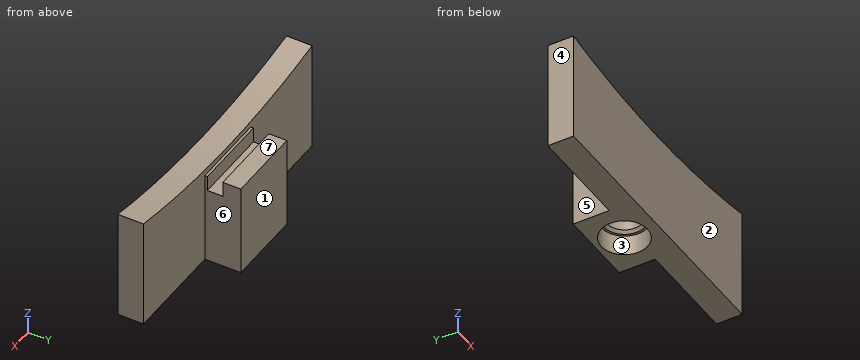
from build123d import *

# Parameters (mm, degrees)
BOSS_EXTRUDE1_DEPTH             = 5
SKETCH4_W                       = 15
SKETCH4_H                       = 18
BOSS_EXTRUDE2_DEPTH             = 0.5
SKETCH5_W                       = 15
SKETCH5_H                       = 15
BOSS_EXTRUDE3_DEPTH             = 3
SKETCH6_W                       = 15
SKETCH6_H                       = 18
BOSS_EXTRUDE4_DEPTH             = 3.5
SKETCH9_R                       = 4.5
CUT_EXTRUDE1_DEPTH              = 4
M8X1_0_TAPPED_HOLE1_D           = 7
M8X1_0_TAPPED_HOLE1_DEPTH       = 8
M8X1_0_TAPPED_HOLE1_CSINK_D     = 8.05
M8X1_0_TAPPED_HOLE1_CSINK_ANGLE = 90
M8X1_0_TAPPED_HOLE1_TIP         = 2.103012167


with BuildPart() as part:
    # Sketch1 → Boss-Extrude1 (new body)
    with BuildSketch(Plane(origin=(0, 0, 0), x_dir=(1, 0, 0), z_dir=(0, 1, 0))):
        with BuildLine():
            Line((0, 9.997621031), (0, 31.54))
            Line((0, 31.54), (55, 31.54))
            Line((55, 31.54), (55, 9.997621031))
            ThreePointArc((55, 9.997621031), (27.5, 12.54), (0, 9.997621031))
        make_face()
    extrude(amount=BOSS_EXTRUDE1_DEPTH)

    # Sketch4 → Boss-Extrude2 (add)
    with BuildSketch(Plane(origin=(0, 5, 0), x_dir=(1, 0, 0), z_dir=(0, 1, 0))):
        with Locations((27.5, 22.54)):
            Rectangle(SKETCH4_W, SKETCH4_H)
    extrude(amount=BOSS_EXTRUDE2_DEPTH)

    # Sketch5 → Boss-Extrude3 (add)
    with BuildSketch(Plane(origin=(0, 5.5, 0), x_dir=(1, 0, 0), z_dir=(0, 1, 0))):
        with Locations((27.5, 24.04)):
            Rectangle(SKETCH5_W, SKETCH5_H)
    extrude(amount=BOSS_EXTRUDE3_DEPTH)

    # Sketch6 → Boss-Extrude4 (add)
    with BuildSketch(Plane(origin=(0, 8.5, 0), x_dir=(1, 0, 0), z_dir=(0, 1, 0))):
        with Locations((27.5, 22.54)):
            Rectangle(SKETCH6_W, SKETCH6_H)
    extrude(amount=BOSS_EXTRUDE4_DEPTH)

    # Sketch9 → Cut-Extrude1 (cut)
    with BuildSketch(Plane(origin=(0, 0, -31.54), x_dir=(-1, 0, 0), z_dir=(0, 0, -1))):
        with Locations((-27.5, 6.5)):
            Circle(SKETCH9_R)
    extrude(amount=-CUT_EXTRUDE1_DEPTH, mode=Mode.SUBTRACT)

    # M8x1.0 Tapped Hole1
    with Locations(Plane(origin=(0, 0, -27.54), x_dir=(-1, 0, 0), z_dir=(0, 0, -1))):
        with Locations((-27.5, 6.5)):
            CounterSinkHole(M8X1_0_TAPPED_HOLE1_D / 2, M8X1_0_TAPPED_HOLE1_CSINK_D / 2, depth=M8X1_0_TAPPED_HOLE1_DEPTH, counter_sink_angle=M8X1_0_TAPPED_HOLE1_CSINK_ANGLE)
            with Locations((0, 0, -(M8X1_0_TAPPED_HOLE1_DEPTH + M8X1_0_TAPPED_HOLE1_TIP / 2))):  # 118° drill point
                Cone(0, M8X1_0_TAPPED_HOLE1_D / 2, M8X1_0_TAPPED_HOLE1_TIP, mode=Mode.SUBTRACT)


solid = part.part
Source: CAD feature listing. Evaluate the final solid. Frame: model axes, mm. Face numbers are marked on the shaded views. A direction names the side the tool comes from. Give positions to 0.01 mm unless a question says otherwise; leave off trailing zeros. Order: outer loops, then holes, each group sorted by start corner. A loop starts at its lowest first (then second) coordinate and runs counter-clockwise, first axis right, second up. Notation, with made-up numbers: (13, -8) -> (39, -8) arc R19 ccw to (39, 18) -> close; hole circle Ø7 at (-16, 7.5). An arc over 180 degrees is marked (long way). Use a Markdown table: item, result.
1) Mould query, pull axis Y, two halves, no side actions, for the marked faces 1, 2, 3 and 4. Classes: +Y half, -Y half, draft (parallel to the pull), parting line (faces both ways), or undercut.
Answer list:
| item | result |
|---|---|
| face 1 | +Y half |
| face 2 | -Y half |
| face 3 | undercut |
| face 4 | draft |
2) Contact query for flat-ended pins moving along their axis: P1, Ø3.5, axis at y = 9, z = -26.5, coming from the +X side; P2, Ø2.5, axis at x = 25.5, y = 6.5, coming from the -Z side; P3, Ø5, axis at x = 16.5, y = 1.5, coming from the +Z side. Output: stop coordinate, or through.
Answer list:
| item | result |
|---|---|
| P1 | x = 35 |
| P2 | z = -19.39 |
| P3 | z = -11.93 |
3) Ray query, line 1 along Y through (x, z) = (27.5, -29.4); line 2 along Y through (x, z) = (27.5, -24.25); line 3 along X through (y, z) = (6.5, -21.75). Return the intervals inside material, ascending. Write a range as [from, to].
Answer list:
| item | result |
|---|---|
| line 1 | [0, 2], [11, 12] |
| line 2 | [0, 3], [10, 12] |
| line 3 | [20, 24], [31, 35] |
4) Section query C-C, the plane x = 48. Return the cut outline in (y, z), then the cut area to 3 significant figures.
Answer list:
| item | result |
|---|---|
| outline | (0, -31.54) -> (5, -31.54) -> (5, -11.13) -> (0, -11.13) -> close |
| area | 102 mm² |
5) Section query B-B, the plane x = 5.5. Return the cut outline in (y, z).
Answer list:
| item | result |
|---|---|
| outline | (0, -31.54) -> (5, -31.54) -> (5, -10.92) -> (0, -10.92) -> close |
6) Reachability of the marked faces 5, 6 and 7 from +Z, -Z, +X, -X, +Y, -Y: full face, straight path, thin tool, end or side. Return the list, or none.
Answer list:
| item | result |
|---|---|
| face 5 | +Z, -Z, -X, +Y |
| face 6 | +Z, -Z, +X, +Y |
| face 7 | +Z, +X, -X, +Y |
7) Section query A-A, the plane z = -23.75. Return the cut outline in (x, y), then the cut area to 3 significant figures.
Answer list:
| item | result |
|---|---|
| outline | (0, 0) -> (55, 0) -> (55, 5) -> (35, 5) -> (35, 12) -> (20, 12) -> (20, 5) -> (0, 5) -> close; hole circle Ø7 at (27.5, 6.5) |
| area | 342 mm² |
